```python
from build123d import *

# Parameters (mm, degrees)
EXTRUDE1_DEPTH = 5.3
SKETCH2_R      = 1.5
EXTRUDE2_DEPTH = 2.3
FILLET1_R      = 1.5
SKETCH3_R      = 0.125
EXTRUDE3_DEPTH = 5.3


with BuildPart() as part:
    # Sketch1 → Extrude1 (new body)
    with BuildSketch(Plane.XY):
        Polygon((-1, 0.5), (1, 0.5), (1.5, 0), (2.05, 0), (2.05, 6.4), (-2.05, 6.4), (-2.05, 0), (-1.5, 0), align=None)
    extrude(amount=-EXTRUDE1_DEPTH)

    # Sketch2 → Extrude2 (add)
    with BuildSketch(Plane.XY):
        with Locations(Location((0, 3, 0), (0, 0, 180))):
            Circle(SKETCH2_R)
    extrude(amount=EXTRUDE2_DEPTH)

    # Fillet1
    fillet1_edges = [part.edges().sort_by_distance(p)[0] for p in [
        (1.5, 3, 2.3),
    ]]
    fillet(fillet1_edges, radius=FILLET1_R)

    # Sketch3 → Extrude3 (add)
    with BuildSketch(Plane.XZ.offset(-0.5)):
        with Locations(Location((1.25, -4, 0), (0, 0, 180))):
            Circle(SKETCH3_R)
        with Locations(Location((-1.25, -4, 0), (0, 0, 90))):
            Circle(SKETCH3_R)
    extrude(amount=EXTRUDE3_DEPTH)


solid = part.part
```
Check sheet for the modelled part. Datum: model origin and axes. Units: mm. Give positions to 0.01 mm unless a question says otherwise; leave off trailing zeros. Write each loop counter-clockwise with the first axis right and the second up, starting at its lowest first coordinate (ties: lowest second). Pieces come first, ordered by that corner, then holes.
Item 1: Cross-section at D-D (x = -1.25). Enter the section's corners in (y, z) (3 decimals), and give its area (3 significant figures).
Item 2: Scan lines: L1, parallel to Z at x = 1.5, y = 3.5; L2, parallel to Y at x = -0.7, z = -1.5; L3, parallel to Y at x = -1.55, z = -1. Record each from-to range of solid material in increasing order.
Item 3: Cross-section at B-B (z = -1.5). Enter the section's corners in (x, y).
Item 4: Gauge pin test, flat end, axial feed: pin 1 (1.5 mm diameter, centred on y = 4, z = 1, fed in from -X). Record the tip position at first contact, or that the pin passes through.
Item 5: Cross-section at C-C (y = -2). Enter the section's corners in (x, z) (3 decimals), and give its area (3 significant figures).
Item 6: Draft check along X on faces 1 (the face through (0, 6.4, -3)), 2 (the face through (0.195, 1.513, 0.394)), 3 (the face through (0, 0.5, -3)). Enter one of: released by +X, released by -X, zero draft, split by the parting line, or undercut.
Item 7: Cross-section at A-A (y = 3). Enter the section's corners in (x, z).
Report:
1. outline: (-4.8, -4.125) - (0.25, -4.125) - (0.25, -5.3) - (6.4, -5.3) - (6.4, 0) - (3.829, 0) - (3.829, 0.8) arc R0.829 ccw to (2.171, 0.8) - (2.171, 0) - (0.25, 0) - (0.25, -3.875) - (-4.8, -3.875) - close
1. area: 36.3 mm2
2. L1: z = -5.3 to 0
2. L2: y = 0.5 to 6.4
2. L3: y = 0 to 6.4
3. outline: (-2.05, 0) - (-1.5, 0) - (-1, 0.5) - (1, 0.5) - (1.5, 0) - (2.05, 0) - (2.05, 6.4) - (-2.05, 6.4) - close
4. pin 1: stops at x = -1.48
5. outline: circle Ø0.25 at (-1.25, -4); circle Ø0.25 at (1.25, -4)
5. area: 0.0982 mm2
6. face 1: zero draft
6. face 2: split by the parting line
6. face 3: undercut
7. outline: (-2.05, -5.3) - (2.05, -5.3) - (2.05, 0) - (1.5, 0) - (1.5, 0.8) arc R1.5 ccw to (-1.5, 0.8) - (-1.5, 0) - (-2.05, 0) - close
